Part model, mm, in its own coordinate system. Face numbers are marked on the shaded views. A direction names the side the tool comes from. Coordinates: 2 decimals unless noted, no trailing zeros. Loops run counter-clockwise (first coordinate to the right, second up) from the corner with the lowest first, then second, coordinate; pieces in that order, holes last. Notation, with made-up numbers: (36, 45) -> (44, 45) arc R20 cw to (44, 62) -> close; hole circle Ø8 at (81.25, 26.5). An arc over 180 degrees is marked (long way). Use one line per item in the form item = value. Start each with the question number.
(1) Band-saw the part on A-A on y = 217. Give the cut face in (x, z).
(2) Drill centre lines: L1, parallel to X at y = 2.7, z = 0; L2, parallel to X at y = 2, z = 18; L3, parallel to Y at x = -13, z = -7. Where is each one in solid material? Low to high. Write a range as [from, to].
(3) 3-axis set-ups, long thin cutter, end or side, ignore diameter. For the marked faces 1 and 2: which of +Z, -Z, +X, -X, +Y, -Y reach the whole face in a straight line?
(4) Pin check, flat tips, straight feed: P1, Ø6, axis at x = -14.5, z = 5.5, coming from the +Y side; P2, Ø8, axis at x = -3.5, y = 73, coming from the -Z side; P3, Ø4.5, axis at x = -18, z = 0, coming from the +Y side. Stop position of each tip, or through.
```python
from build123d import *

# Parameters (mm, degrees)
SKETCH_1_R          = 22.5
SKETCH_1_R_2        = 1.65
EXTRUDE_1_DEPTH     = 4
SKETCH_2_R          = 7.5
EXTRUDE_2_DEPTH     = 320
SKETCH_3_R          = 1.4
CUT_EXTRUDE_1_DEPTH = 10
CHAMFER_1_SIZE      = 6


with BuildPart() as part:
    # 草图1 → 凸台-拉伸1 (new body)
    with BuildSketch(Plane(origin=(0, 0, 0), x_dir=(1, 0, 0), z_dir=(0, 1, 0))):
        with Locations(Location((0, 0, 0), (0, 0, 270))):
            Circle(SKETCH_1_R)
        with Locations(Location((-18, 0, 0), (0, 0, 270))):
            Circle(SKETCH_1_R_2, mode=Mode.SUBTRACT)
        with Locations(Location((18, 0, 0), (0, 0, 270))):
            Circle(SKETCH_1_R_2, mode=Mode.SUBTRACT)
        with Locations(Location((0, 18, 0), (0, 0, 270))):
            Circle(SKETCH_1_R_2, mode=Mode.SUBTRACT)
        with Locations(Location((0, -18, 0), (0, 0, 270))):
            Circle(SKETCH_1_R_2, mode=Mode.SUBTRACT)
    extrude(amount=EXTRUDE_1_DEPTH)

    # 草图2 → 凸台-拉伸2 (add)
    with BuildSketch(Plane(origin=(0, 4, 0), x_dir=(1, 0, 0), z_dir=(0, 1, 0))):
        with Locations(Location((0, 0, 0), (0, 0, 270))):
            Circle(SKETCH_2_R)
    extrude(amount=EXTRUDE_2_DEPTH)

    # 草图3 → 切除-拉伸1 (cut)
    with BuildSketch(Plane(origin=(0, 324, 0), x_dir=(1, 0, 0), z_dir=(0, 1, 0))):
        with Locations(Location((0, 0, 0), (0, 0, 270))):
            Circle(SKETCH_3_R)
    extrude(amount=-CUT_EXTRUDE_1_DEPTH, mode=Mode.SUBTRACT)

    # 倒角1
    chamfer_1_edges = [part.edges().sort_by_distance(p)[0] for p in [
        (0, 4, -7.5),
    ]]
    chamfer(chamfer_1_edges, length=CHAMFER_1_SIZE)


solid = part.part
```
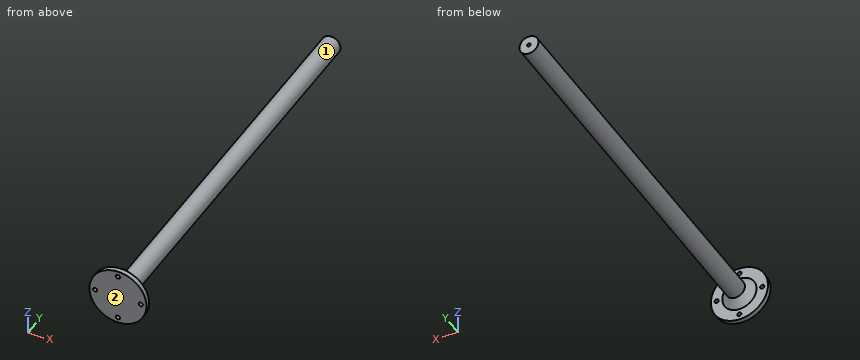
A:
q1.outline = circle Ø15 at (0, 0)
q2.L1 = [-22.5, -19.65], [-16.35, 16.35], [19.65, 22.5]
q2.L2 = [-13.5, -1.65], [1.65, 13.5]
q2.L3 = [0, 4]
q3.face_1 = +Y
q3.face_2 = +Z, -Z, +X, -X, -Y
q4.P1 = 4.99
q4.P2 = -7.5
q4.P3 = 4
